Here's how the part is built. I have some questions about the finished solid (model axes, mm). Face numbers are marked on the shaded views. A direction names the side the tool comes from. Round coordinates to 2 decimals unless told otherwise and drop trailing zeros. Write each loop counter-clockwise with the first axis right and the second up, starting at its lowest first coordinate (ties: lowest second). Pieces come first, ordered by that corner, then holes. Notation, with made-up numbers: (-27.5, 11) -> (-20.5, 11) arc R17 ccw to (-20.5, 16) -> close; hole circle Ø6 at (32.25, 60.5). An arc over 180 degrees is marked (long way). Answer as CSV lines item,"result".
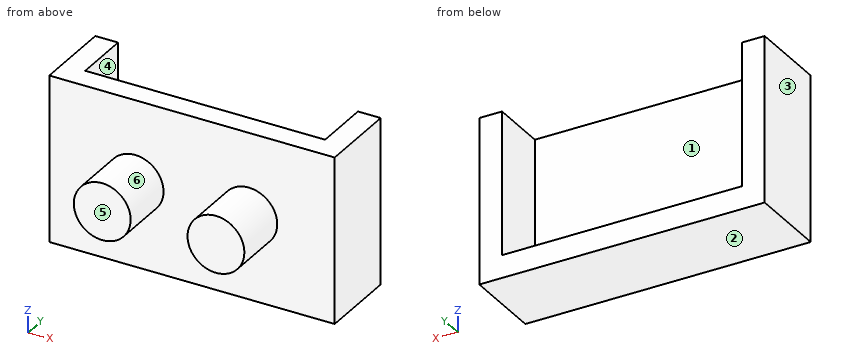
from build123d import *

# Parameters (mm, degrees)
BOSS_EXTRUDE1_DEPTH = 5
SKETCH1_3_W         = 21.1
SKETCH1_3_H         = 12.6
BOSS_EXTRUDE2_DEPTH = 2
SKETCH3_R           = 2.5
BOSS_EXTRUDE4_DEPTH = 5


with BuildPart() as part:
    # Sketch1 → Boss-Extrude1 (new body)
    with BuildSketch(Plane(origin=(0, 0, 0), x_dir=(1, 0, 0), z_dir=(0, 1, 0))):
        Polygon((23.1, 14.6), (-2, 14.6), (-2, 0), (0, 0), (0, 12.6), (21.1, 12.6), (21.1, 0), (23.1, 0), align=None)
    extrude(amount=BOSS_EXTRUDE1_DEPTH)

    # Sketch1_3 → Boss-Extrude2 (add)
    with BuildSketch(Plane(origin=(0, 0, 0), x_dir=(1, 0, 0), z_dir=(0, 1, 0))):
        with Locations((10.55, 6.3)):
            Rectangle(SKETCH1_3_W, SKETCH1_3_H)
        Polygon((23.1, 14.6), (-2, 14.6), (-2, 0), (0, 0), (0, 12.6), (21.1, 12.6), (21.1, 0), (23.1, 0), align=None)
    extrude(amount=-BOSS_EXTRUDE2_DEPTH)

    # Sketch3 → Boss-Extrude4 (add)
    with BuildSketch(Plane.XZ.offset(2)):
        with Locations(Location((5.55, -7.3, 0), (0, 0, 90))):
            Circle(SKETCH3_R)
        with Locations(Location((15.55, -7.3, 0), (0, 0, 90))):
            Circle(SKETCH3_R)
    extrude(amount=BOSS_EXTRUDE4_DEPTH)


solid = part.part
Item 1: Will this pin go through, and if not, where does the flat tip stop? pin 1 (2.5 mm diameter, centred on x = 9, y = 3.5, fed in from +Z).
Results found:
pin 1,"stops at z = -12.6"
Item 2: Suppose I cut it at C-C, the plane y = -3.5. List the corners of the cut face in (x, z) for me, then the cut area to 3 significant figures.
Results found:
outline,"circle Ø5 at (5.55, -7.3); circle Ø5 at (15.55, -7.3)"
area,"39.3 mm²"
Item 3: Suppose I cut it at B-B, the plane x = 15.55. List the corners of the cut face in (y, z) for me, then the cut area to 3 significant figures.
Results found:
outline,"(-7, -9.8) -> (-2, -9.8) -> (-2, -14.6) -> (5, -14.6) -> (5, -12.6) -> (0, -12.6) -> (0, 0) -> (-2, 0) -> (-2, -4.8) -> (-7, -4.8) -> close"
area,"64.2 mm²"
Item 4: If we mould it in two halves opening along X, with no side actions, what happens to the marked faces 1, 2 and 3? For each: pulls with the +X half, pulls with the -X half, needs draft (parallel to the pull), parting line crosses it, or undercut.
Results found:
face 1,"undercut"
face 2,"needs draft"
face 3,"pulls with the -X half"
Item 5: Suppose I cut it at A-A, the plane y = 3. List the corners of the cut face in (x, z) for me.
Results found:
outline,"(-2, -14.6) -> (23.1, -14.6) -> (23.1, 0) -> (21.1, 0) -> (21.1, -12.6) -> (0, -12.6) -> (0, 0) -> (-2, 0) -> close"
Item 6: I need wall thicknesses on L1, parallel to X at y = 1, z = -2.25; L2, parallel to Y at x = 15, z = -7.75; L3, parallel to Y at x = 3.25, z = -5.25. Which ranges of each line are inside material? Lowest first, please.
Results found:
L1,"x = -2 to 0, 21.1 to 23.1"
L2,"y = -7 to 0"
L3,"y = -2 to 0"
Item 7: Suppose I cut it at D-D, the plane z = -7.3. List the corners of the cut face in (x, y) for me.
Results found:
outline,"(-2, -2) -> (3.05, -2) -> (3.05, -7) -> (8.05, -7) -> (8.05, -2) -> (13.05, -2) -> (13.05, -7) -> (18.05, -7) -> (18.05, -2) -> (23.1, -2) -> (23.1, 5) -> (21.1, 5) -> (21.1, 0) -> (0, 0) -> (0, 5) -> (-2, 5) -> close"
Item 8: For the marked faces 4, 5 and 6, which set-ups out of +Z, -Z, +X, -X, +Y, -Y let a thin tool reach every point of the face, with its end or its side?
Results found:
face 4,"+Z, +Y"
face 5,"+Z, -Z, +X, -X, -Y"
face 6,"-Y"
